Build history of the part. All positions in model axes, mm. Face numbers are marked on the shaded views. A direction names the side the tool comes from. Coordinates: 2 decimals unless noted, no trailing zeros. Write each loop counter-clockwise with the first axis right and the second up, starting at its lowest first coordinate (ties: lowest second). Pieces come first, ordered by that corner, then holes. Notation, with made-up numbers: (50.5, 55) -> (60.5, 55) arc R24 ccw to (60.5, 90) -> close; hole circle Ø3 at (1, 62.25). An arc over 180 degrees is marked (long way). Write each question's results on one line, items separated by ' | '. Start each with the question number.
Q1. Saw through at A-A on x = -16. Give the cut face in (y, z), and give its area (3 significant figures).
Q2. Drill centre lines: line 1 (Z direction, x = -59.5, y = -25); line 2 (Y direction, x = -54.5, z = -43.5); line 3 (Z direction, x = -75.5, y = 1). Where is each one in solid material? Low to high.
Q3. Saw through at C-C on y = -30. Give the cut face in (x, z).
Q4. Drop flat-ended pins along their axis: pin 1 Ø12 at (x, z) = (-65, -34) entering from -Y; pin 2 Ø22.5 at (x, y) = (-40, -21) entering from +Z; pin 3 Ø6 at (y, z) = (-3.5, -51) entering from +X. Give the stop position or say it passes through.
Q5. Tool access for the marked faces 1 and 2: list every direction of +Z, -Z, +X, -X, +Y, -Y with a clear straight run to the whole face (end or side of a thin tool).
Q6. Saw through at B-B on z = -14. Give the cut face in (x, y).
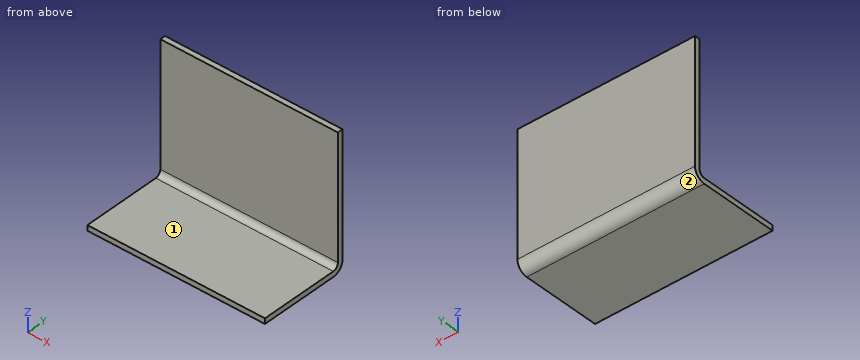
Autodesk Inventor part; units mm, degrees
ref_plane "YZ Plane" through (0, 0, 0) normal (1, 0, 0) x (0, 1, 0)
ref_plane "XZ Plane" through (0, 0, 0) normal (0, 1, 0) x (-1, 0, 0)
ref_plane "XY Plane" through (0, 0, 0) normal (0, 0, 1) x (1, 0, 0)
sketch "Sketch1" plane through (0, 0, 0) normal (0, 1, 0) x (-1, 0, 0)
  line L0 (0, 0) -> (101.6, 0)
  line L1 (101.6, 0) -> (101.6, -76.2)
  line L2 (101.6, -76.2) -> (0, -76.2)
  line L3 (0, -76.2) -> (0, 0)
  dimension "d0" = 101.6
  dimension "d1" = 76.2
extrude "Plate1" add sketch "Sketch1" along normal blind 3.048
sketch "Sketch2" plane through (0, 3.048, -73.152) normal (0, 0, -1) x (-1, 0, 0)
  line L0 (101.6, 0) -> (0, 0)
  line L1 (0, 0) -> (0, -50.8)
  line L2 (0, -50.8) -> (101.6, -50.8)
  line L3 (101.6, -50.8) -> (101.6, 0)
edge flange "Flange1" height 50.8 angle 90 thickness 3.048 bend radius 3.048 thickness toward (0, 0, -1) relief tear relief width 3.048 relief depth 1.524 edges at (-50.8, 0, -76.2) wall of the first edge with corners at (-101.6, 3.048, -73.152) (0, 3.048, -73.152) (0, -47.752, -73.152) (-101.6, -47.752, -73.152)
bend "Bend1"
corner "Corner1"
equation "\"d3\" = BendReliefWidth"
equation "\"d4\" = BendReliefDepth"
equation "\"d5\" = MinimumRemnant"
equation "\"d6\" = BendRadius"
equation "\"d9\" = BendRadius"
equation "\"d10\" = CornerReliefSize"
equation "\"d11\" = GapSize"
equation "\"d12\" = JacobiRadiusSize"
equation "\"BendRadius\" = Thickness"
equation "\"BendReliefWidth\" = Thickness"
equation "\"BendReliefDepth\" = 0.5 * Thickness"
equation "\"CornerReliefSize\" = 4 * Thickness"
equation "\"MinimumRemnant\" = 2 * Thickness"
equation "\"TransitionRadius\" = BendRadius"
equation "\"JacobiRadiusSize\" = BendRadius"
equation "\"GapSize\" = Thickness"
equation "\"d2\" = BendRadius"
properties part number "motorBracket"
Returned:
1) outline: (-47.75, -76.2) -> (-3.05, -76.2) arc R6.1 ccw to (3.05, -70.1) -> (3.05, 0) -> (0, 0) -> (0, -70.1) arc R3.05 cw to (-3.05, -73.15) -> (-47.75, -73.15) -> close | area: 372 mm2
2) line 1: z = -76.2 to -73.15 | line 2: y = 0 to 3.05 | line 3: z = -74.66 to 0
3) outline: (-101.6, -76.2) -> (0, -76.2) -> (0, -73.15) -> (-101.6, -73.15) -> close
4) pin 1: stops at y = 0 | pin 2: stops at z = -73.15 | pin 3: passes through
5) face 1: +Z, +X, -X, -Y | face 2: -Z, +X, -X, +Y
6) outline: (-101.6, 0) -> (0, 0) -> (0, 3.05) -> (-101.6, 3.05) -> close
